```python
from build123d import *

# Parameters (mm, degrees)
SKETCH1_W           = 5
SKETCH1_H           = 10
BOSS_EXTRUDE1_DEPTH = 4
FILLET2_R           = 4
FILLET4_R           = 2


with BuildPart() as part:
    # Sketch1 → Boss-Extrude1 (new body)
    with BuildSketch(Plane(origin=(0, 0, 0), x_dir=(0, 0, -1), z_dir=(1, 0, 0))):
        Polygon((-46.5, -15), (-46.5, -20.025618734), (-34.5, -20.025618734), (-34.5, -15), (-24.5, -15), (-24.5, -20.025618734), (-12.5, -20.025618734), (-12.5, -15), (29.5, -15), (29.5, -20.025618734), (41.5, -20.025618734), (41.5, -15), (51.5, -15), (49, -5), (-8.333333333, -5), (-10, 15), (-49, 15), (-51.5, -15), align=None)
        with Locations((-22, 0)):
            Rectangle(SKETCH1_W, SKETCH1_H, mode=Mode.SUBTRACT)
        with Locations((-37, 0)):
            Rectangle(SKETCH1_W, SKETCH1_H, mode=Mode.SUBTRACT)
    extrude(amount=BOSS_EXTRUDE1_DEPTH)

    # Fillet2
    fillet2_edges = [part.edges().sort_by_distance(p)[0] for p in [
        (2, 15, 49),
        (2, 15, 10),
        (2, -5, 8.333333333),
        (2, -5, -49),
    ]]
    fillet(fillet2_edges, radius=FILLET2_R)

    # Fillet4
    fillet4_edges = [part.edges().sort_by_distance(p)[0] for p in [
        (2, -15, 51.5),
        (2, -15, -51.5),
    ]]
    fillet(fillet4_edges, radius=FILLET4_R)


solid = part.part
```
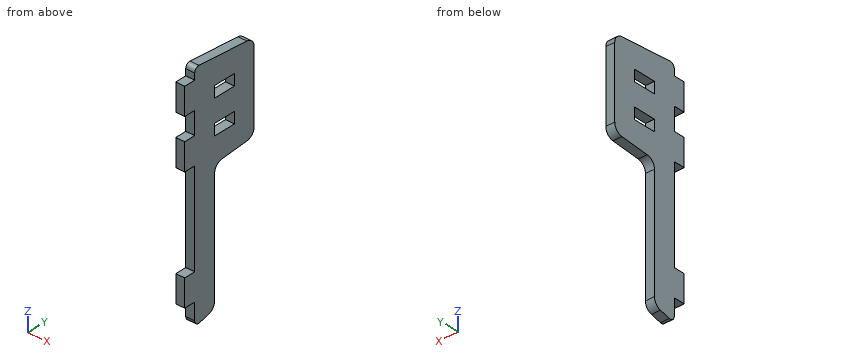
For this review, take the finished solid that the model builds, in its own axes (mm). Give positions to 0.01 mm unless a question says otherwise; leave off trailing zeros. Loops run counter-clockwise (first coordinate to the right, second up) from the corner with the lowest first, then second, coordinate; pieces in that order, holes last. Notation, with made-up numbers: M 11,-36 L 59,-36 A30 cw 59,1 Z; hole C -34,1.5 d1. An arc over 180 degrees is marked long. One line per item, written item: value. Start each with the question number.
Q1. Add section D-D (z = -13.5). Give the boundary of the cut face in (x, y), and give its area (3 significant figures).
Q2. Add section B-B (y = -17). Give the boundary of the cut face in (x, z), and give its area (3 significant figures).
Q3. Add section A-A (x = 2.9). Count the separate pieces of the cut face and the enclosed holes in it, and give its area (3 significant figures).
Q4. For L1, parallel to Z at x = 2, y = -16; L2, parallel to Y at x = 3.3, z = 38.5; L3, parallel to Z at x = 2.2, y = -2, list the stretches that pass through material, from the lowest coordinate up.
Q5. Clearance check with flat-ended pins moving along their axes: pin 1 Ø1.5 at (x, y) = (1, 0.5) entering from +Z; pin 2 Ø2 at (x, y) = (2.5, -18.5) entering from -Z; pin 3 Ø2 at (x, z) = (2, -47) entering from -Y. State where each tip first meets the part, or that it passes through.
Q6. Add section C-C (z = 29.5). Give the boundary of the cut face in (x, y).
Reply:
1. outline: M 0,-15 L 4,-15 L 4,-5 L 0,-5 Z
1. area: 40.0 mm²
2. outline: M 0,-41.5 L 4,-41.5 L 4,-29.5 L 0,-29.5 Z; M 0,12.5 L 4,12.5 L 4,24.5 L 0,24.5 Z; M 0,34.5 L 4,34.5 L 4,46.5 L 0,46.5 Z
2. area: 144 mm²
3. separate pieces: 1
3. enclosed holes: 2
3. area: 1,900 mm²
4. L1: -41.5 to -29.5, 12.5 to 24.5, 34.5 to 46.5
4. L2: -20.03 to -5, 5 to 15
4. L3: 8.53 to 19.5, 24.5 to 34.5, 39.5 to 50.42
5. pin 1: z = 50.27
5. pin 2: z = -41.5
5. pin 3: y = -15
6. outline: M 0,-15 L 4,-15 L 4,15 L 0,15 Z
